Verification items for the finished model (mm, model axes). Give positions to 0.01 mm unless a question says otherwise; leave off trailing zeros. Order: outer loops, then holes, each group sorted by start corner. A loop starts at its lowest first (then second) coordinate and runs counter-clockwise, first axis right, second up. Notation, with made-up numbers: (40, 23) -> (92, 23) arc R19 cw to (92, 48) -> close; hole circle Ø1 at (-19, -7). An arc over 180 degrees is marked (long way). Return JSON: item names as keys, results as strings. Group by question number.
(1) Cross-section at A-A on x = 60.95. Enter the section's corners in (y, z).
(2) Cross-section at C-C on x = 84.5. Enter the section's corners in (y, z), then the cut area to 3 significant figures.
(3) Cross-section at B-B on z = -4.25. State how many separate pieces and enclosed holes the cut face has, then the cut area to 3 significant figures.
(4) Depth check by flat-ended pin: pin 1 Ø1.5 at (y, z) = (-0.5, -5) entering from +X. Enter the tip coordinate at first touch or a pass-through.
(5) Thickness scan on line 1 along Y through (x, z) = (23.05, -6.5); line 2 along Y through (x, z) = (-11, -6.5); line 3 along X through (y, z) = (5.5, -8.75). Record the ranges inside material, lowest first.
from build123d import *

# Parameters (mm, degrees)
SKETCH7_W           = 170
SKETCH7_H           = 100
BOSS_EXTRUDE1_DEPTH = 10
SKETCH1_R           = 2
CUT_EXTRUDE2_DEPTH  = 131.384048104
LPATTERN1_COUNT     = 4
LPATTERN1_PITCH     = 28
SKETCH8_W           = 134.95
SKETCH8_H           = 41
CUT_EXTRUDE3_DEPTH  = 131.384048104


with BuildPart() as part:
    # Sketch7 → Boss-Extrude1 (new body)
    with BuildSketch(Plane.XY):
        with Locations((35, 0)):
            Rectangle(SKETCH7_W, SKETCH7_H)
    extrude(amount=-BOSS_EXTRUDE1_DEPTH)

    # Sketch1 → Cut-Extrude2 (cut, through all)
    with BuildSketch(Plane.XY):
        with Locations((4.95, -24.3)):
            Circle(SKETCH1_R)
        with Locations(Location((-4.95, -24.3, 0), (0, 0, 180))):
            Circle(SKETCH1_R)
        with Locations((-4.95, 24.3)):
            Circle(SKETCH1_R)
        with Locations(Location((4.95, 24.3, 0), (0, 0, 180))):
            Circle(SKETCH1_R)
    cut_extrude2 = extrude(amount=-CUT_EXTRUDE2_DEPTH, mode=Mode.SUBTRACT)

    # LPattern1: Cut-Extrude2 ×4
    with Locations(*[(i * LPATTERN1_PITCH, 0, 0) for i in range(1, LPATTERN1_COUNT)]):
        add(cut_extrude2, mode=Mode.SUBTRACT)

    # Sketch8 → Cut-Extrude3 (cut, through all)
    with BuildSketch(Plane.XY):
        with Locations((52.525, 0)):
            Rectangle(SKETCH8_W, SKETCH8_H)
    extrude(amount=-CUT_EXTRUDE3_DEPTH, mode=Mode.SUBTRACT)


solid = part.part
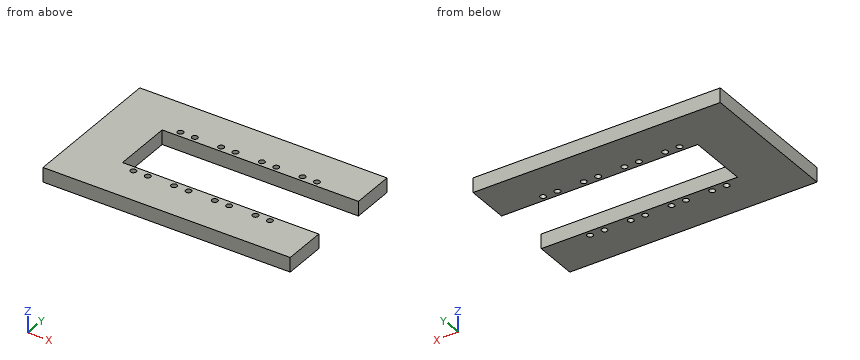
Verdict:
{
 "1": {"outline": "(-50, -10) -> (-26.3, -10) -> (-26.3, 0) -> (-50, 0) -> close; (-22.3, -10) -> (-20.5, -10) -> (-20.5, 0) -> (-22.3, 0) -> close; (20.5, -10) -> (22.3, -10) -> (22.3, 0) -> (20.5, 0) -> close; (26.3, -10) -> (50, -10) -> (50, 0) -> (26.3, 0) -> close"},
 "2": {"outline": "(-50, -10) -> (-20.5, -10) -> (-20.5, 0) -> (-50, 0) -> close; (20.5, -10) -> (50, -10) -> (50, 0) -> (20.5, 0) -> close", "area": "590 mm²"},
 "3": {"separate pieces": "1", "enclosed holes": "16", "area": "11,300 mm²"},
 "4": {"pin 1": "x = -14.95"},
 "5": {"line 1": "-50 to -26.3, -22.3 to -20.5, 20.5 to 22.3, 26.3 to 50", "line 2": "-50 to -20.5, 20.5 to 50", "line 3": "-50 to -14.95"}
}
